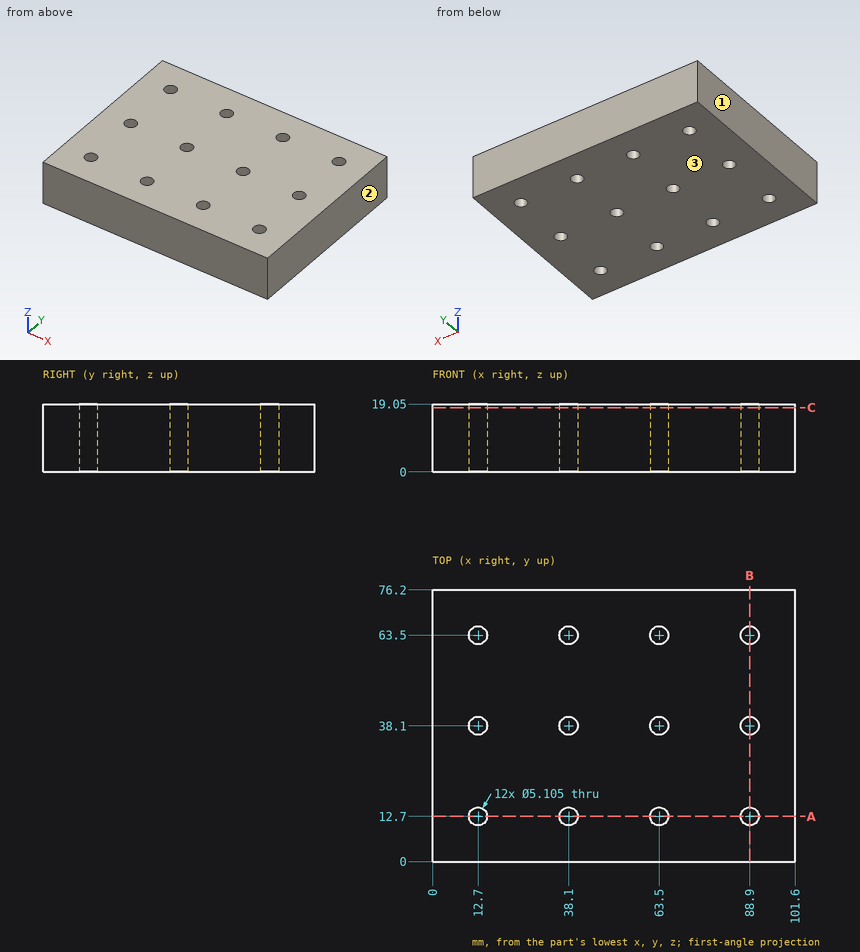
Geometry check sheet. Reference: drawing and pictorial views, mm from the part's lowest x, y, z. Round coordinates to 2 decimals unless told otherwise and drop trailing zeros. Loops run counter-clockwise (first coordinate to the right, second up) from the corner with the lowest first, then second, coordinate; pieces in that order, holes last. Notation, with made-up numbers: (-12.5, -39.5) - (17.5, -39.5) arc R14 cw to (17.5, -14.5) - close; hole circle Ø5 at (-27.5, 27). An arc over 180 degrees is marked (long way). One line per question, with ' | ' between items. Start each with the question number.
1. Cross-section at C-C on z = 18. State how many separate pieces and enclosed holes the cut face has, then the cut area to 3 significant figures.
2. Draft check along X on the marked faces 1, 2 and 3. Enter one of: released by +X, released by -X, zero draft, split by the parting line, or undercut.
3. Cross-section at B-B on x = 88.9. Record the cut outline in (y, z), then the cut area to 3 significant figures.
4. Cross-section at A-A on y = 12.7. Record the cut outline in (x, z).
5. Scan lines: line 1 (Y direction, x = 63.5, z = 11.75); line 2 (X direction, y = 62.5, z = 15); line 3 (X direction, y = 39.5, z = 2.5) (1 decimal). Record each from-to range of solid material in increasing order. Write a range as [from, to].
Taken from the geometry:
1) separate pieces: 1 | enclosed holes: 12 | area: 7,500 mm²
2) face 1: released by -X | face 2: released by +X | face 3: zero draft
3) outline: (0, 0) - (10.15, 0) - (10.15, 19.05) - (0, 19.05) - close; (15.25, 0) - (35.55, 0) - (35.55, 19.05) - (15.25, 19.05) - close; (40.65, 0) - (60.95, 0) - (60.95, 19.05) - (40.65, 19.05) - close; (66.05, 0) - (76.2, 0) - (76.2, 19.05) - (66.05, 19.05) - close | area: 1,160 mm²
4) outline: (0, 0) - (10.15, 0) - (10.15, 19.05) - (0, 19.05) - close; (15.25, 0) - (35.55, 0) - (35.55, 19.05) - (15.25, 19.05) - close; (40.65, 0) - (60.95, 0) - (60.95, 19.05) - (40.65, 19.05) - close; (66.05, 0) - (86.35, 0) - (86.35, 19.05) - (66.05, 19.05) - close; (91.45, 0) - (101.6, 0) - (101.6, 19.05) - (91.45, 19.05) - close
5) line 1: [0, 10.15], [15.25, 35.55], [40.65, 60.95], [66.05, 76.2] | line 2: [0, 10.35], [15.05, 35.75], [40.45, 61.15], [65.85, 86.55], [91.25, 101.6] | line 3: [0, 10.6], [14.8, 36], [40.2, 61.4], [65.6, 86.8], [91, 101.6]
